Geometry check sheet. Reference: the model listing, model coordinates, mm. Give positions to 0.01 mm unless a question says otherwise; leave off trailing zeros. Write each loop counter-clockwise with the first axis right and the second up, starting at its lowest first coordinate (ties: lowest second). Pieces come first, ordered by that corner, then holes. Notation, with made-up numbers: (-32, 62) - (-27, 62) arc R12 cw to (-27, 76) - close; hole circle Ø4 at (0.5, -15). An arc over 180 degrees is marked (long way). One line per question, with ' | ' between items. Start each with the question number.
Q1. Gauge pin test, flat end, axial feed: P1, Ø1.5, axis at x = -2.5, z = -12, coming from the +Y side. Record the tip position at first contact, or that the pin passes through.
Q2. Section check D-D on y = 2. Record the boundary of the cut face in (x, z).
Q3. Section check A-A on z = 19. Record the boundary of the cut face in (x, y), and give its area (3 significant figures).
Q4. Thickness scan on L1, parallel to Y at x = 0, z = 7; L2, parallel to Y at x = -0.25, z = 7. Record the ranges inside material, lowest first. Write a range as [from, to].
Q5. Section check B-B on x = 1. Record the boundary of the cut face in (y, z).
Q6. Section check C-C on y = -0.75. Record the boundary of the cut face in (x, z).
Q7. Release check for a two-part mould opening along X. For faces 1 (the face through (-1.5, -0.07, -0.35)), 2 (the face through (-2.98, -1.255, -0.35)), 3 (the face through (0, -2, -25)), 4 (the face through (1.255, -2.98, -0.35)) record: +X half, -X half, draft (parallel to the pull), parting line (faces both ways), or undercut.
Autodesk Inventor part; units mm, degrees
sketch "Skizze1" plane through (0, 0, 0) normal (0, 0, 1) x (1, 0, 0)
  line L0 (0, 4.9) -> (0, -4.9)
  line L1 (-4.9, 0) -> (4.9, 0)
  line L2 (0, 3.5) -> (2.4749, 2.4749)
  line L3 (2.4749, 2.4749) -> (3.5, 0)
  line L4 (3.5, 0) -> (2.4749, -2.4749)
  line L5 (2.4749, -2.4749) -> (0, -3.5)
  line L6 (0, -3.5) -> (-2.4749, -2.4749)
  line L7 (-2.4749, -2.4749) -> (-3.5, 0)
  line L8 (-3.5, 0) -> (-2.4749, 2.4749)
  line L9 (-2.4749, 2.4749) -> (0, 3.5)
  circle A0 centre (0, 0) radius 1.5
  dimension "d0" = 3
extrude "Extrusion1" add sketch "Skizze1" along normal mid plane 50 contours L2 L3 L1 A0 L0 | L0 A0 L1 L8 L9 | L1 L4 L5 L0 A0 | A0 L0 L6 L7 L1
properties part number "StutzeHinten"
Working result:
1) P1: stops at y = 2.78
2) outline: (-2.67, -25) - (2.67, -25) - (2.67, 25) - (-2.67, 25) - close
3) outline: (-3.5, 0) - (-2.47, -2.47) - (0, -3.5) - (2.47, -2.47) - (3.5, 0) - (2.47, 2.47) - (0, 3.5) - (-2.47, 2.47) - close; hole circle Ø3 at (0, 0) | area: 27.6 mm2
4) L1: y = [-3.5, -1.5], [1.5, 3.5] | L2: y = [-3.4, -1.48], [1.48, 3.4]
5) outline: (-3.09, -25) - (-1.12, -25) - (-1.12, 25) - (-3.09, 25) - close; (1.12, -25) - (3.09, -25) - (3.09, 25) - (1.12, 25) - close
6) outline: (-3.19, -25) - (-1.3, -25) - (-1.3, 25) - (-3.19, 25) - close; (1.3, -25) - (3.19, -25) - (3.19, 25) - (1.3, 25) - close
7) face 1: undercut | face 2: -X half | face 3: draft | face 4: +X half
